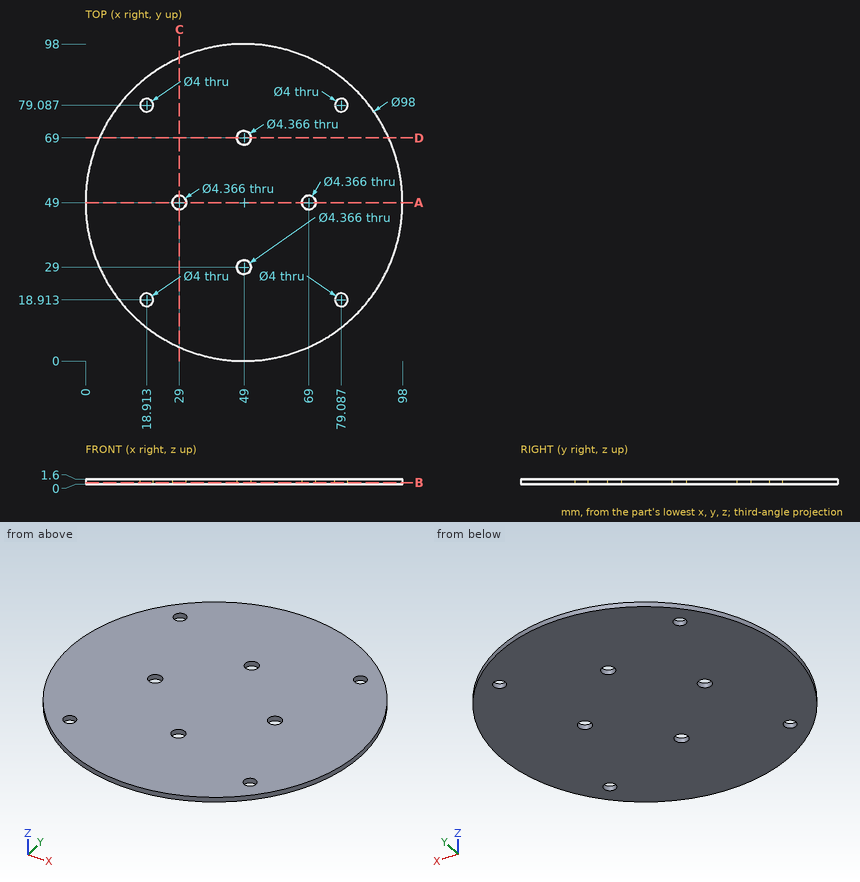
Study the drawing (mm; zero at the part's minimum x, y, z) and answer. Coordinates: 2 decimals unless noted, no trailing zeros. Loops run counter-clockwise (first coordinate to the right, second up) from the corner with the lowest first, then second, coordinate; pieces in that order, holes last. Notation, with made-up numbers: M 64.5,14.25 L 92.5,14.25 A12 cw 92.5,26.25 Z; hole C 18.5,82.5 d1. An arc over 180 degrees is marked long. Answer in a Markdown table with one row per item.
1) Find section A-A (y = 49). Determine the outline of the cut face in (x, z).
Answers below:
| item | result |
|---|---|
| outline | M 0,0 L 26.82,0 L 26.82,1.6 L 0,1.6 Z; M 31.18,0 L 66.82,0 L 66.82,1.6 L 31.18,1.6 Z; M 71.18,0 L 98,0 L 98,1.6 L 71.18,1.6 Z |
2) Given pin 1 (2.5 mm diameter, centred on x = 49, y = 29, fed in from +Z), flat-ended and moving along its own axis, determine where the tip first touches the part or whether it passes through.
Answers below:
| item | result |
|---|---|
| pin 1 | through |
3) Find section B-B (z = 0.45). Count the separate pieces of the cut face and the enclosed holes in it, then the cut area to 3 significant figures.
Answers below:
| item | result |
|---|---|
| separate pieces | 1 |
| enclosed holes | 8 |
| area | 7,430 mm^2 |
4) Find section C-C (x = 29). Determine the outline of the cut face in (y, z).
Answers below:
| item | result |
|---|---|
| outline | M 4.27,0 L 46.82,0 L 46.82,1.6 L 4.27,1.6 Z; M 51.18,0 L 93.73,0 L 93.73,1.6 L 51.18,1.6 Z |
5) Find the intervals of material crossed by probe 1 along Y at (x, z) = (49, 1.2); probe 2 along X at (y, z) = (20.5, 0.9) (1 decimal); probe 3 along Y at (x, z) = (19, 1.2) (1 decimal), in increasing order.
Answers below:
| item | result |
|---|---|
| probe 1 | 0 to 26.82, 31.18 to 66.82, 71.18 to 98 |
| probe 2 | 9.1 to 17.7, 20.1 to 77.9, 80.3 to 88.9 |
| probe 3 | 10.3 to 16.9, 20.9 to 77.1, 81.1 to 87.7 |
